Part model, mm, in its own coordinate system. Round coordinates to 2 decimals unless told otherwise and drop trailing zeros. Loops run counter-clockwise (first coordinate to the right, second up) from the corner with the lowest first, then second, coordinate; pieces in that order, holes last. Notation, with made-up numbers: M 84.25,77.25 L 142.25,77.25 A26 cw 142.25,92.25 Z; hole C -14,76 d10. An arc over 180 degrees is marked long. Put each result on its own line as item: value. Start each with the question number.
1) Pull direction Y, two halves, no side cores. Call faces 1 (the flat face through (6, -70, 0)), 2 (the cylindrical face through (27.358, -90.638, 1.521)), 3 (the cylindrical face through (-13.668, -58.785, 1.521)), 4 (the flat face through (7, -142, 1)): +Y half, -Y half, draft (parallel to the pull), parting line (faces both ways), or undercut.
2) Probe line 1 along Y through (x, z) = (26.5, 1.45); line 2 along X through (y, z) = (-136.65, 0.8); line 3 along Y through (x, z) = (20, 0.95). List the from-to ranges inside material, lowest first.
3) Slice it at C-C on z = 1.5. State how many separate pieces and enclosed holes the cut face has, then the cut area to 3 significant figures.
4) Drop a flat-ended pin along its axis: pin 1 Ø5 at (x, y) = (5, -136.65) entering from -Z. Give the stop position or say it passes through.
5) Slice it at B-B on x = 5. Give the cut face in (y, z), then the cut area to 3 significant figures.
6) Slice it at A-A on y = -136.65. Give the cut face in (x, z).
Autodesk Inventor part; units mm, degrees
ref_plane "YZ Plane" through (0, 0, 0) normal (1, 0, 0) x (0, 1, 0)
ref_plane "XZ Plane" through (0, 0, 0) normal (0, 1, 0) x (-1, 0, 0)
ref_plane "XY Plane" through (0, 0, 0) normal (0, 0, 1) x (1, 0, 0)
sketch "Sketch1" plane through (0, 0, 0) normal (0, 0, 1) x (1, 0, 0)
  line L0 (0, 0) -> (25, 0)
  line L1 (25, 0) -> (25, -142)
  line L2 (25, -142) -> (0, -142)
  line L3 (0, -142) -> (0, 0)
  line L4 (20, -5.35) -> (5, -5.35) construction
  line L5 (5, -5.35) -> (5, -136.65) construction
  line L6 (5, -136.65) -> (20, -136.65) construction
  line L7 (20, -136.65) -> (20, -5.35) construction
  circle A0 centre (20, -5.35) radius 2.794
  circle A1 centre (5, -5.35) radius 2.794
  circle A2 centre (20, -136.65) radius 2.794
  circle A3 centre (5, -136.65) radius 2.794
  line L8 (0, 0) -> (-24, 0)
  line L9 (-24, 0) -> (-24, -142)
  line L10 (-24, -142) -> (0, -142)
  line L11 (25, -142) -> (37, -142)
  line L12 (37, -142) -> (37, 0)
  line L13 (37, 0) -> (25, 0)
  point P0 (20, -71)
  point P1 (25, -71)
  point P2 (12.5, -136.65)
  point P3 (12.5, -142)
  dimension "d0" = 142
  dimension "d1" = 25
  dimension "d2" = 131.3
  dimension "d3" = 15
  dimension "d4" = 5.588
  dimension "d7" = 12
  dimension "d8" = 24
extrude "Extrusion1" add sketch "Sketch1" along normal blind 3
sketch "Sketch2" plane through (0, 0, 3) normal (0, 0, 1) x (1, 0, 0)
  line L0 (26.3967, -88.79) -> (-13.3967, -88.79) construction
  line L1 (-13.3967, -88.79) -> (-13.3967, -60.85) construction
  line L2 (-13.3967, -60.85) -> (26.3967, -60.85) construction
  line L3 (26.3967, -60.85) -> (26.3967, -88.79) construction
  line L4 (-24, -142) -> (37, -142) construction
  circle A0 centre (26.3967, -60.85) radius 2.0828
  circle A1 centre (26.3967, -88.79) radius 2.0828
  circle A2 centre (-13.3967, -60.85) radius 2.0828
  circle A3 centre (-13.3967, -88.79) radius 2.0828
  point P0 (0, 0)
  point P1 (6.5, -88.79)
  point P2 (6.5, -142)
  dimension "d9" = 53.21
  dimension "d10" = 27.94
  dimension "d11" = 39.7933
  dimension "d12" = 4.1656
extrude "Extrusion2" cut sketch "Sketch2" against normal blind 3
properties part number "Watercooler_Mounting_Plate"
Recorded:
1. face 1: draft
1. face 2: undercut
1. face 3: undercut
1. face 4: -Y half
2. line 1: y = -142 to -90.87, -86.71 to -62.93, -58.77 to 0
2. line 2: x = -24 to 2.21, 7.79 to 17.21, 22.79 to 37
2. line 3: y = -142 to -139.44, -133.86 to -8.14, -2.56 to 0
3. separate pieces: 1
3. enclosed holes: 8
3. area: 8,510 mm2
4. pin 1: passes through
5. outline: M -142,0 L -139.44,0 L -139.44,3 L -142,3 Z; M -133.86,0 L -8.14,0 L -8.14,3 L -133.86,3 Z; M -2.56,0 L 0,0 L 0,3 L -2.56,3 Z
5. area: 392 mm2
6. outline: M -24,0 L 2.21,0 L 2.21,3 L -24,3 Z; M 7.79,0 L 17.21,0 L 17.21,3 L 7.79,3 Z; M 22.79,0 L 37,0 L 37,3 L 22.79,3 Z
